Input: part model. Units: mm. Frame: model coordinates. A direction names the side the tool comes from. Round coordinates to 2 decimals unless told otherwise and drop trailing zeros. Write each loop counter-clockwise with the first axis right and the second up, starting at its lowest first coordinate (ties: lowest second). Pieces come first, ordered by that corner, then holes. Notation, with made-up numbers: (84, 54) -> (135, 54) arc R25 cw to (135, 79) -> close; hole circle Ø6 at (32.25, 56). An arc over 180 degrees is marked (long way). Write item = value, one per line. Start each with the question number.
```python
from build123d import *

# Parameters (mm, degrees)
F0_R        = 15.6
F0_R_2      = 14
F0_R_3      = 2
F1_DEPTH    = 3
F2_DEPTH    = 20
F3_R        = 1.5
F4_R        = 1
F5_R        = 2
F6_DEPTH    = 3
F7_T1_DEPTH = 3


# Not quite as in the source:
# - a fillet or chamfer that OpenCascade refuses, or shapes differently, is made with other operations: its cross-section is extruded or revolved along the edge and cut away or added


with BuildPart() as f1:
    # F0 (on Top) → F1 (new body)
    with BuildSketch(Plane.XY):
        Circle(F0_R)
        Circle(F0_R_2, mode=Mode.SUBTRACT)
        Circle(F0_R_2)
        Circle(F0_R_3, mode=Mode.SUBTRACT)
        Circle(F0_R_3)
    extrude(amount=F1_DEPTH)

    # F0 (on Top) → F2 (join)
    with BuildSketch(Plane.XY):
        Circle(F0_R)
        Circle(F0_R_2, mode=Mode.SUBTRACT)
    extrude(amount=F2_DEPTH)

    # F3
    f3_edges = [f1.edges().sort_by_distance(p)[0] for p in [
        (-15.6, 0, 0),
    ]]
    fillet(f3_edges, radius=F3_R)

    # F4
    f4_edges = [f1.edges().sort_by_distance(p)[0] for p in [
        (-14, 0, 20),
    ]]
    fillet(f4_edges, radius=F4_R)

    # F5 (on face) + F0 (on Top) → F6 (cut, through all)
    with BuildSketch(Plane.XY):
        with BuildLine():
            add(Edge.make_bspline(
                [(0, -2.5137708586), (0, -4.1458795261), (-1.7837920859, -8.9341028845), (-10.8913647651, -3.867257191), (-4.0863468312, 3.7691965699), (0, 8.5115667947)],
                knots=[0, 0, 0, 0, 0.2681845993, 0.5480579368, 1, 1, 1, 1], degree=3))
            add(Edge.make_bspline(
                [(0, -2.5137708586), (0, -4.1458795261), (1.7837920859, -8.9341028845), (10.8913647651, -3.867257191), (4.0863468312, 3.7691965699), (0, 8.5115667947)],
                knots=[0, 0, 0, 0, 0.2681845993, 0.5480579368, 1, 1, 1, 1], degree=3))
        make_face()
        Circle(F5_R, mode=Mode.SUBTRACT)
    with BuildSketch(Plane.XY):
        Circle(F0_R_3)
    extrude(amount=F6_DEPTH, mode=Mode.SUBTRACT)

    # F7: fillet of radius 0.4 on 1 edges, made by hand

    # F7_s2 → F7_t1 (cut)
    with BuildSketch(Plane.XY):
        with BuildLine():
            ThreePointArc((0.3762881855, -4.5548185088), (0, -4.2904916507), (-0.3762881855, -4.5548185088))
            Line((-0.3762881855, -4.5548185088), (-0.3838139492, -4.5521050459))
            ThreePointArc((-0.3838139492, -4.5521050459), (-0.1103093457, -3.5489845707), (-0.008, -2.5137708586))
            Line((-0.008, -2.5137708586), (0.008, -2.5137708586))
            ThreePointArc((0.008, -2.5137708586), (0.1103093457, -3.5489845707), (0.3838139492, -4.5521050459))
            Line((0.3838139492, -4.5521050459), (0.3762881855, -4.5548185088))
        make_face()
    extrude(amount=F7_T1_DEPTH, mode=Mode.SUBTRACT)


solid = f1.part
```
1. Reachability of faces 4 (the cylindrical face through (12.932, -5.362, 10.888)), 5 (the flat face through (0, -6, 0)) from +Z, -Z, +X, -X, +Y, -Y: full face, straight path, thin tool, end or side. Return the list, or none.
2. Line query: line 1 along Y through (x, z) = (0, 14.5); line 2 along Y through (x, z) = (-2.5, 18.5); line 3 along Z through (x, y) = (12, 4.5). Output: solid intervals per line, ascending.
3. Pin query (flat end, axial travel): P1, Ø10, axis at y = -9.5, z = 6, coming from the +X side; P2, Ø4, axis at x = 5.5, y = 1, coming from the +Z side; P3, Ø10, axis at y = 8, z = 3, coming from the -X side. Return the tip coordinate at first contact, or that it passes through.
4. Mould query, pull axis Y, two halves, no side actions, for faces 1 (the flat face through (-8, 13, 20)), 2 (the flat face through (0, -6, 3)), 3 (the cylindrical face through (-11.5, 10.54, 10.62)). Classes: pulls with the +Y half, pulls with the -Y half, needs draft (parallel to the pull), parting line crosses it, or undercut.
5. Section A-A (z = 3.5). Output: boundary loops of the cut face in (x, y), then the cut area to 3 significant figures.
Check sheet entries:
q1.face_4 = +Z
q1.face_5 = -Z, +X, -X, +Y, -Y
q2.line_1 = -15.6 to -14, 14 to 15.6
q2.line_2 = -15.4 to -13.77, 13.77 to 15.4
q2.line_3 = 0 to 3
q3.P1 = 14.94
q3.P2 = 3
q3.P3 = -15.31
q4.face_1 = needs draft
q4.face_2 = undercut
q4.face_3 = parting line crosses it
q5.outline = circle Ø31.2 at (0, 0); hole circle Ø28 at (0, 0)
q5.area = 149 mm2
